Source: CAD feature listing. Evaluate the final solid. Frame: model axes, mm. Round coordinates to 2 decimals unless told otherwise and drop trailing zeros. Write each loop counter-clockwise with the first axis right and the second up, starting at its lowest first coordinate (ties: lowest second). Pieces come first, ordered by that corner, then holes. Notation, with made-up numbers: M -1,-25 L 37,-25 A25 ccw 37,11 Z; hole C 53.25,9 d1. An arc over 180 degrees is marked long. Answer in a Markdown table with one row per item. Add a question column.
Item 1: Material intervals for probe 1 along Z at (x, y) = (-2, 0.1); probe 2 along X at (y, z) = (-0.3, 0.7); probe 3 along Z at (x, y) = (-9, 0.65), sorted ascending.
Item 2: Cut plane A-A on x = -8. Return loops of the section in (y, z).
Item 3: Cut plane B-B on x = -16. Return loops of the section in (y, z), and give its area (3 significant figures).
Item 4: Contact query for a flat-ended pin moving along its axis: pin 1 (1 mm diameter, centred on x = 3, y = 0.5, fed in from +Z). Output: stop coordinate, or through.
from build123d import *

# Parameters (mm, degrees)
F1_R       = 0.9
F3_R       = 0.8
F2_FACE_R  = 0.1
F2_FACE1_R = 0.1


with BuildPart() as f2:
    # F2: sweep along a path in F0
    with BuildLine(Plane.XY) as f2_path:
        Line((-10, 0), (0, 0))
    # F1 (on Right) → F2 (sweep)
    with BuildSketch(Plane.YZ):
        Circle(F1_R)
    sweep(path=f2_path.line)

    # F3
    f3_edges = [f2.edges().sort_by_distance(p)[0] for p in [
        (0, -0.9, 0),
        (-10, -0.9, 0),
    ]]
    fillet(f3_edges, radius=F3_R)

    # F5: sweep along a path in F4
    with BuildLine(Plane.XY) as f5_path:
        Line((0, 0), (15, 0))
    # F2_face (on face) → F5 (sweep)
    with BuildSketch(Plane.YZ):
        Circle(F2_FACE_R)
    sweep(path=f5_path.line)

    # F7: sweep along a path in F6
    with BuildLine(Plane.XY) as f7_path:
        Line((-10, 0), (-25, 0))
    # F2_face1 (on face) → F7 (sweep)
    with BuildSketch(Plane(origin=(-10, 0, 0), x_dir=(0, -1, 0), z_dir=(-1, 0, 0))):
        Circle(F2_FACE1_R)
    sweep(path=f7_path.line)


solid = f2.part
Results below:
| question | item | result |
|---|---|---|
| 1 | probe 1 | -0.89 to 0.89 |
| 1 | probe 2 | -9.65 to -0.35 |
| 1 | probe 3 | -0.62 to 0.62 |
| 2 | outline | C 0,0 d1.8 |
| 3 | outline | C 0,0 d0.2 |
| 3 | area | 0.0314 mm2 |
| 4 | pin 1 | z = 0.1 |
